Verification items for the finished model (mm, model axes). Face numbers are marked on the shaded views. A direction names the side the tool comes from. Round coordinates to 2 decimals unless told otherwise and drop trailing zeros. Order: outer loops, then holes, each group sorted by start corner. A loop starts at its lowest first (then second) coordinate and runs counter-clockwise, first axis right, second up. Notation, with made-up numbers: M 9,68 L 63,68 A16 cw 63,95 Z; hole C 61,-5 d1. An arc over 180 degrees is marked long. Use one line per item in the form item = value. Start each with the question number.
Item 1: Cross-section at B-B on z = -17.5. Enter the section's corners in (x, y).
Item 2: Cross-section at D-D on y = 18.5. Enter the section's corners in (x, z).
Item 3: Cross-section at A-A on y = 37. Enter the section's corners in (x, z), then the cut area to 3 significant figures.
Item 4: Go/stop test with flat-tipped pins: pin 1 Ø3 at (x, y) = (42, 56) entering from +Z; pin 2 Ø12 at (x, z) = (19, -58) entering from +Y. Record where each tip stops, or that it passes through.
Item 5: Thickness scan on probe 1 along Y at (x, z) = (17, -4); probe 2 along X at (y, z) = (44, -34.5); probe 3 along Y at (x, z) = (47.5, -43). Record the ranges inside material, lowest first. Write a range as [from, to].
Item 6: Tool access check on the marked faces 1, 2 and 3. Record the directions out of +Z, -Z, +X, -X, +Y, -Y that give a thin tool (end or side, any length) a straight path to the whole face; none if there is none.
from build123d import *

# Parameters (mm, degrees)
SALIENTE_EXTRUIR1_DEPTH = 30
SALIENTE_EXTRUIR2_DEPTH = 20
SALIENTE_EXTRUIR3_DEPTH = 15
SALIENTE_EXTRUIR4_DEPTH = 1


with BuildPart() as part:
    # Croquis1 → Saliente-Extruir1 (new body)
    with BuildSketch(Plane(origin=(0, 0, 0), x_dir=(1, 0, 0), z_dir=(0, 1, 0))):
        with BuildLine():
            Line((10, 0), (60, 0))
            ThreePointArc((60, 0), (67.071067812, 2.928932188), (70, 10))
            Line((70, 10), (70, 60))
            ThreePointArc((70, 60), (67.071067812, 67.071067812), (60, 70))
            Line((60, 70), (10, 70))
            ThreePointArc((10, 70), (2.928932188, 67.071067812), (0, 60))
            Line((0, 60), (0, 10))
            ThreePointArc((0, 10), (2.928932188, 2.928932188), (10, 0))
        make_face()
    extrude(amount=SALIENTE_EXTRUIR1_DEPTH)

    # Croquis2 → Saliente-Extruir2 (add)
    with BuildSketch(Plane(origin=(0, 30, 0), x_dir=(1, 0, 0), z_dir=(0, 1, 0))):
        with BuildLine():
            Line((10, 0), (59.904487732, 0))
            ThreePointArc((59.904487732, 0), (66.975555544, 2.928932188), (69.904487732, 10))
            Line((69.904487732, 10), (69.904487732, 60.022676449))
            ThreePointArc((69.904487732, 60.022676449), (66.975555544, 67.093744261), (59.904487732, 70.022676449))
            Line((59.904487732, 70.022676449), (10, 70.022676449))
            ThreePointArc((10, 70.022676449), (2.928932188, 67.093744261), (0, 60.022676449))
            Line((0, 60.022676449), (0, 10))
            ThreePointArc((0, 10), (2.928932188, 2.928932188), (10, 0))
        make_face()
    extrude(amount=SALIENTE_EXTRUIR2_DEPTH)

    # Croquis3 → Saliente-Extruir3 (add)
    with BuildSketch(Plane(origin=(0, 50, 0), x_dir=(1, 0, 0), z_dir=(0, 1, 0))):
        with BuildLine():
            ThreePointArc((45.714988655, 45.583878221), (35.109068959, 49.985918595), (24.503149262, 45.583878221))
            Line((24.503149262, 45.583878221), (35.109068959, 35.008376267))
            Line((35.109068959, 35.008376267), (45.714988655, 45.583878221))
        make_face()
        with BuildLine():
            Line((35.109068959, 35.008376267), (24.503149262, 45.583878221))
            ThreePointArc((24.503149262, 45.583878221), (20.131526631, 35.008376267), (24.503149262, 24.432874313))
            Line((24.503149262, 24.432874313), (35.109068959, 35.008376267))
        make_face()
        with BuildLine():
            Line((45.714988655, 45.583878221), (35.109068959, 35.008376267))
            Line((35.109068959, 35.008376267), (45.714988655, 24.432874313))
            ThreePointArc((45.714988655, 24.432874313), (48.950625688, 29.286656114), (50.086611287, 35.008376267))
            ThreePointArc((50.086611287, 35.008376267), (48.950625688, 40.730096419), (45.714988655, 45.583878221))
        make_face()
        with BuildLine():
            Line((45.714988655, 24.432874313), (35.109068959, 35.008376267))
            Line((35.109068959, 35.008376267), (24.503149262, 24.432874313))
            ThreePointArc((24.503149262, 24.432874313), (35.109068959, 20.030833939), (45.714988655, 24.432874313))
        make_face()
    extrude(amount=SALIENTE_EXTRUIR3_DEPTH)

    # Croquis4 → Saliente-Extruir4 (add)
    with BuildSketch(Plane(origin=(0, 65, 0), x_dir=(1, 0, 0), z_dir=(0, 1, 0))):
        with BuildLine():
            ThreePointArc((26.040054757, 25.966127976), (35.178980063, 22.173048991), (44.317905369, 25.966127976))
            Line((44.317905369, 25.966127976), (35.178980063, 35.079108201))
            Line((35.178980063, 35.079108201), (26.040054757, 25.966127976))
        make_face()
        with BuildLine():
            Line((35.178980063, 35.079108201), (44.317905369, 25.966127976))
            ThreePointArc((44.317905369, 25.966127976), (47.106131346, 30.148649135), (48.085039273, 35.079108201))
            ThreePointArc((48.085039273, 35.079108201), (47.106131346, 40.009567268), (44.317905369, 44.192088426))
            Line((44.317905369, 44.192088426), (35.178980063, 35.079108201))
        make_face()
        with BuildLine():
            Line((26.040054757, 25.966127976), (35.178980063, 35.079108201))
            Line((35.178980063, 35.079108201), (26.040054757, 44.192088426))
            ThreePointArc((26.040054757, 44.192088426), (22.272920853, 35.079108201), (26.040054757, 25.966127976))
        make_face()
        with BuildLine():
            Line((26.040054757, 44.192088426), (35.178980063, 35.079108201))
            Line((35.178980063, 35.079108201), (44.317905369, 44.192088426))
            ThreePointArc((44.317905369, 44.192088426), (35.178980063, 47.985167411), (26.040054757, 44.192088426))
        make_face()
    extrude(amount=SALIENTE_EXTRUIR4_DEPTH)


solid = part.part
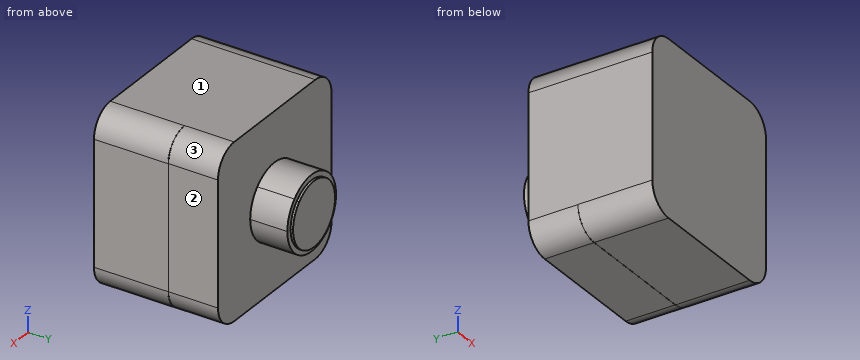
Output values:
q1.outline = M 0,0 L 70,0 L 70,30 L 69.9,30 L 69.9,50 L 0,50 Z
q2.outline = M 0,-60 A10 ccw 10,-70 L 60,-70 A10 ccw 70,-60 L 70,-10 A10 ccw 60,0 L 10,0 A10 ccw 0,-10 Z
q3.outline = M 0,-60.02 A10 ccw 10,-70.02 L 59.9,-70.02 A10 ccw 69.9,-60.02 L 69.9,-10 A10 ccw 59.9,0 L 10,0 A10 ccw 0,-10 Z
q3.area = 4,810 mm2
q4.pin_1 = -21.03
q4.pin_2 = 50
q5.probe_1 = [0, 50]
q5.probe_2 = [0, 69.9]
q5.probe_3 = [0, 65]
q6.face_1 = +Z, +X, -X, +Y, -Y
q6.face_2 = +Z, -Z, +X, +Y
q6.face_3 = +Z, +X, +Y
